from build123d import *

# Parameters (mm, degrees)
F0_R     = 10.3251
F1_DEPTH = 7.9375
F2_R     = 6.35
F3_R     = 9.92251
F4_DEPTH = 7.9375
F6_R     = 12.7
F7_R     = 4.7625


with BuildPart() as f1:
    # F0 (on Top) → F1 (new body)
    with BuildSketch(Plane.XY):
        with BuildLine():
            Line((-53.975, -22.225), (0, -22.225))
            ThreePointArc((0, -22.225), (22.225, 0), (0, 22.225))
            Line((0, 22.225), (-53.975, 22.225))
            Line((-53.975, 22.225), (-53.975, 44.45))
            Line((-53.975, 44.45), (-111.125, 44.45))
            Line((-111.125, 44.45), (-111.125, -44.45))
            Line((-111.125, -44.45), (-53.975, -44.45))
            Line((-53.975, -44.45), (-53.975, -22.225))
        make_face()
        with Locations((-38.1, 0)):
            Circle(F0_R, mode=Mode.SUBTRACT)
        Circle(F0_R, mode=Mode.SUBTRACT)
    extrude(amount=F1_DEPTH)

    # F2
    f2_edges = [f1.edges().sort_by_distance(p)[0] for p in [
        (-53.975, -22.225, 3.96875),
        (-53.975, 22.225, 3.96875),
    ]]
    fillet(f2_edges, radius=F2_R)

    # F3 (on face) → F4 (join)
    with BuildSketch(Plane.XZ.offset(44.45)):
        with BuildLine():
            Line((-111.125, 44.45), (-111.125, 7.9375))
            Line((-111.125, 7.9375), (-53.975, 7.9375))
            Line((-53.975, 7.9375), (-53.975, 44.45))
            ThreePointArc((-53.975, 44.45), (-82.55, 73.025), (-111.125, 44.45))
        make_face()
        with Locations((-82.55, 44.45)):
            Circle(F3_R, mode=Mode.SUBTRACT)
    extrude(amount=-F4_DEPTH)

    # F5: F1 across plane


with BuildPart() as f1_1:
    add(f1.part)
    add(f1.part.mirror(Plane.XZ))

    # F6
    f6_edges = [f1_1.edges().sort_by_distance(p)[0] for p in [
        (-82.55, 44.45, 0),
        (-82.55, -44.45, 0),
    ]]
    fillet(f6_edges, radius=F6_R)

    # F7
    f7_edges = [f1_1.edges().sort_by_distance(p)[0] for p in [
        (-82.55, 36.5125, 73.025),
        (-82.55, -36.5125, 73.025),
    ]]
    fillet(f7_edges, radius=F7_R)


solid = f1_1.part
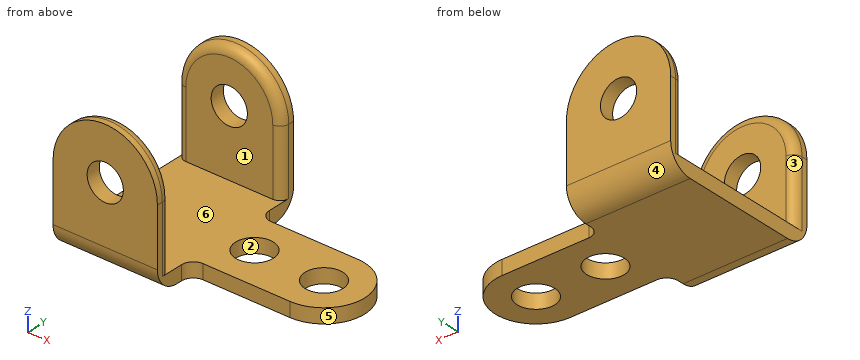
Could you check a few things on this model? Use its own coordinates, in mm. Face numbers are marked on the shaded views. A direction names the side the tool comes from. Round coordinates to 2 decimals unless told otherwise and drop trailing zeros. Order: outer loops, then holes, each group sorted by start corner. A loop starts at its lowest first (then second) coordinate and runs counter-clockwise, first axis right, second up.
Q1. Imagine slicing it at C-C, the plane y = 0. List the corners of the cut face in (x, z) for me (1 decimal).
Geometry says:
outline: (-111.1, 0) - (-48.4, 0) - (-48.4, 7.9) - (-111.1, 7.9) - close; (-27.8, 0) - (-10.3, 0) - (-10.3, 7.9) - (-27.8, 7.9) - close; (10.3, 0) - (22.2, 0) - (22.2, 7.9) - (10.3, 7.9) - close
Q2. Thinking about a two-plate mould opening in Y: for the marked faces 4, 5 and 6, which applies, released by +Y, released by -Y, zero draft, split by the parting line, or undercut?
Geometry says:
face 4: released by +Y
face 5: split by the parting line
face 6: undercut
Q3. I'm going to push flat-ended pins straight in: P1, Ø18.5, axis at x = 0, y = 0, coming from the +Z side; P2, Ø5, axis at y = 40.5, z = 14.5, coming from the +X side (3 decimals); P3, Ø8, axis at x = -90, y = 19, coming from the +Z side; P4, Ø6.5, axis at x = -21, z = 5.5, coming from the -Y side (3 decimals). Where does each tip first touch, or does it pass through?
Geometry says:
P1: passes through
P2: stops at x = -53.975
P3: stops at z = 7.94
P4: stops at y = -22.225
Q4. Imagine slicing it at D-D, the plane z = 41.5. State how many separate pieces and enclosed holes the cut face has, then the cut area to 3 significant figures.
Geometry says:
separate pieces: 4
enclosed holes: 0
area: 587 mm2
Q5. Imagine slicing it at A-A, the plane x = -38.1. List the corners of the cut face in (y, z) for me (1 decimal), then the cut area to 3 significant figures.
Geometry says:
outline: (-22.2, 0) - (-10.3, 0) - (-10.3, 7.9) - (-22.2, 7.9) - close; (10.3, 0) - (22.2, 0) - (22.2, 7.9) - (10.3, 7.9) - close
area: 189 mm2
Q6. Which directions (+Z, -Z, +X, -X, +Y, -Y) give clear straight access to the entire face, cutting with the end or side of a thin tool? Please do the marked faces 1, 2 and 3.
Geometry says:
face 1: +Z, +X, -X
face 2: +Z, -Z
face 3: +Z, -X
Q7. Please list where these lines run through material, in increasing order: probe 1 along Y at (x, z) = (0, 4) (3 decimals); probe 2 along Y at (x, z) = (-72.5, 48.5); probe 3 along Z at (x, y) = (-11.5, 17.5).
Geometry says:
probe 1: y = -22.225 to -10.325, 10.325 to 22.225
probe 2: y = -44.45 to -36.51, 36.51 to 44.45
probe 3: z = 0 to 7.94
